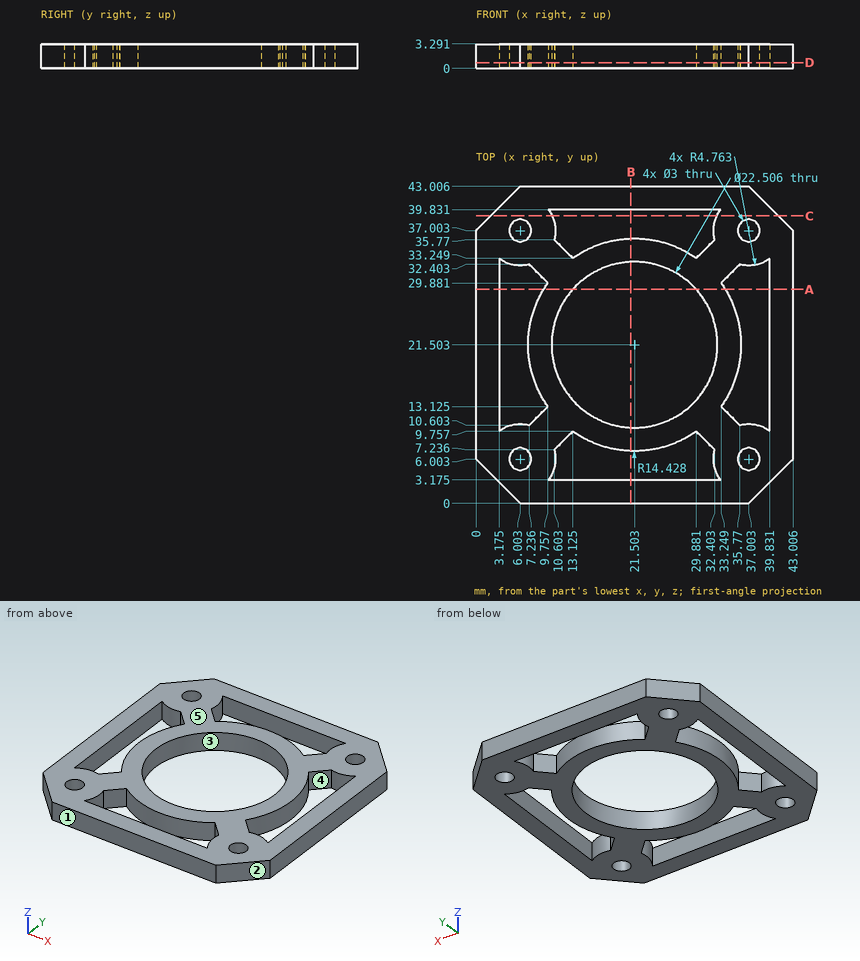
Could you check a few things on this drawing? It's one solid part, dimensions in mm from its lowest x, y, z. A direction names the side the tool comes from. Coordinates: 2 decimals unless noted, no trailing zeros. Write each loop counter-clockwise with the first axis right and the second up, starting at its lowest first coordinate (ties: lowest second). Pieces come first, ordered by that corner, then holes.
Q1. Imagine slicing it at A-A, the plane y = 29. List the corners of the cut face in (x, z) for me (1 decimal).
Results found:
outline: (0, 0) - (3.2, 0) - (3.2, 3.3) - (0, 3.3) - close; (9.2, 0) - (13.1, 0) - (13.1, 3.3) - (9.2, 3.3) - close; (29.9, 0) - (33.8, 0) - (33.8, 3.3) - (29.9, 3.3) - close; (39.8, 0) - (43, 0) - (43, 3.3) - (39.8, 3.3) - close
Q2. Which directions (+Z, -Z, +X, -X, +Y, -Y) give clear straight access to the entire face, cutting with the end or side of a thin tool? Please do the marked faces 4 and 5.
Results found:
face 4: +Z, -Z
face 5: +Z, +X, -X, +Y, -Y
Q3. Please list where these lines run through material, in increasing order: L1, parallel to Y at x = 21, z = 0.3 (1 decimal); L2, parallel to X at y = 31.5, z = 0.5 (1 decimal); L3, parallel to Y at x = 18, z = 0.8 (1 decimal).
Results found:
L1: y = 0 to 3.2, 7.1 to 10.3, 32.7 to 35.9, 39.8 to 43
L2: x = 0 to 3.2, 8.1 to 16.3, 26.7 to 34.9, 39.8 to 43
L3: y = 0 to 3.2, 7.5 to 10.8, 32.2 to 35.5, 39.8 to 43
Q4. For P1, Ø1.8, axis at x = 37, y = 6, coming from the +Z side, with a flat end and sliding along its axis, tell me the tip position at first contact or that it passes through.
Results found:
P1: passes through
Q5. Imagine slicing it at B-B, the plane x = 21. List the corners of the cut face in (y, z) for me (1 decimal).
Results found:
outline: (0, 0) - (3.2, 0) - (3.2, 3.3) - (0, 3.3) - close; (7.1, 0) - (10.3, 0) - (10.3, 3.3) - (7.1, 3.3) - close; (32.7, 0) - (35.9, 0) - (35.9, 3.3) - (32.7, 3.3) - close; (39.8, 0) - (43, 0) - (43, 3.3) - (39.8, 3.3) - close
Q6. Imagine slicing it at C-C, the plane y = 39. List the corners of the cut face in (x, z) for me.
Results found:
outline: (2, 0) - (10.33, 0) - (10.33, 3.29) - (2, 3.29) - close; (32.68, 0) - (41.01, 0) - (41.01, 3.29) - (32.68, 3.29) - close
Q7. If we mould it in two halves opening along X, with no side actions, what happens to the marked faces 1, 2 and 3? For each: +X half, -X half, draft (parallel to the pull), parting line (faces both ways), or undercut.
Results found:
face 1: draft
face 2: +X half
face 3: undercut
Q8. Imagine slicing it at D-D, the plane z = 0.75. Count the separate pieces of the cut face and the enclosed holes in it.
Results found:
separate pieces: 1
enclosed holes: 9
